Design review of the part built by this model. Coordinates are the model's own, in mm. A direction names the side the tool comes from. Coordinates: 2 decimals unless noted, no trailing zeros. Loops run counter-clockwise (first coordinate to the right, second up) from the corner with the lowest first, then second, coordinate; pieces in that order, holes last.
Q1. For P1, Ø5, axis at y = 1.5, z = 13.5, coming from the +X side; P2, Ø2, axis at x = -50, z = 12, coming from the -Y side, all flat-tipped, find the tip position at first contact; note any pin that passes through.
Q2. Add section C-C on y = 0. Give the boundary of the cut face in (x, z) (3 decimals).
Q3. Add section A-A on x = -50.8. Give the boundary of the cut face in (y, z) (3 decimals), and give its area (3 significant figures).
Q4. Machinability: for faces 5 (the face through (-1, 0, 0)), 6 (the face through (82.6, 1.5, 9.9)), which of the approach directions +Z, -Z, +X, -X, +Y, -Y give a long, thin tool a straight path to every point of the face, cutting with its end or side? Answer none if there is none.
Q5. Add section B-B on z = 12.7. Give the boundary of the cut face in (x, y) (3 decimals).
Q6. Wall thickness on probe 1 along Z at (x, y) = (-76.2, 0) (3 decimals); probe 2 along X at (y, z) = (-6, 15); probe 3 along X at (y, z) = (-7.5, 15.25): over which ranges is each line inside the solid? List them lowest first.
Q7. Draft analysis for pull direction X (two halves, no side actions). For faces 1 (the face through (-73.17, -0.18, 13.65)), 2 (the face through (88.9, 3, 15)), 3 (the face through (-53.97, -0.18, 12.84)), 4 (the face through (-1, 12.7, 13)), state which applies: released by +X, released by -X, zero draft, split by the parting line, or undercut.
```python
from build123d import *

# Parameters (mm, degrees)
F0_W     = 177.8
F0_H     = 25.4
F1_DEPTH = 25.4
F2_R     = 3.175
F3_DEPTH = 25.4
F4_R     = 3.175
F5_DEPTH = 12.7


with BuildPart() as f1:
    # F0 (on Top) → F1 (new body)
    with BuildSketch(Plane.XY):
        Rectangle(F0_W, F0_H)
    extrude(amount=F1_DEPTH)

    # F2 (on face) → F3 (cut)
    with BuildSketch(Plane.XZ.offset(12.7)):
        with Locations((-76.2, 12.7)):
            Circle(F2_R)
        with Locations((-50.8, 12.7)):
            Circle(F2_R)
    extrude(amount=-F3_DEPTH, mode=Mode.SUBTRACT)

    # F4 (on face) → F5 (cut)
    with BuildSketch(Plane.YZ.offset(88.9)):
        with Locations((0, 12.7)):
            Circle(F4_R)
    extrude(amount=-F5_DEPTH, mode=Mode.SUBTRACT)


solid = f1.part
```
Entries:
1. P1: stops at x = 88.9
1. P2: passes through
2. outline: (-88.9, 0) - (88.9, 0) - (88.9, 9.525) - (76.2, 9.525) - (76.2, 15.875) - (88.9, 15.875) - (88.9, 25.4) - (-88.9, 25.4) - close; hole circle Ø6.35 at (-76.2, 12.7); hole circle Ø6.35 at (-50.8, 12.7)
3. outline: (-12.7, 0) - (12.7, 0) - (12.7, 9.525) - (-12.7, 9.525) - close; (-12.7, 15.875) - (12.7, 15.875) - (12.7, 25.4) - (-12.7, 25.4) - close
3. area: 484 mm2
4. face 5: -Z, +X, -X, +Y, -Y
4. face 6: +X
5. outline: (-88.9, -12.7) - (-79.375, -12.7) - (-79.375, 12.7) - (-88.9, 12.7) - close; (-73.025, -12.7) - (-53.975, -12.7) - (-53.975, 12.7) - (-73.025, 12.7) - close; (-47.625, -12.7) - (88.9, -12.7) - (88.9, -3.175) - (76.2, -3.175) - (76.2, 3.175) - (88.9, 3.175) - (88.9, 12.7) - (-47.625, 12.7) - close
6. probe 1: z = 0 to 9.525, 15.875 to 25.4
6. probe 2: x = -88.9 to -78.39, -74.01 to -52.99, -48.61 to 88.9
6. probe 3: x = -88.9 to -78.09, -74.31 to -52.69, -48.91 to 88.9
7. face 1: undercut
7. face 2: released by +X
7. face 3: undercut
7. face 4: zero draft
